Design review of the part built by this model. Coordinates are the model's own, in mm. Round coordinates to 2 decimals unless told otherwise and drop trailing zeros. Order: outer loops, then holes, each group sorted by start corner. A loop starts at its lowest first (then second) coordinate and runs counter-clockwise, first axis right, second up. Notation, with made-up numbers: M 51,81 L 85,81 A20 ccw 85,96 Z; hole C 76.5,-32 d9. An arc over 180 degrees is marked long. Use a Markdown table: item, result. Add a question column.
(1) Take a section at C-C (y = -57.48). Write out the cut boundary in (x, z), then the cut area to 3 significant figures.
(2) Take a section at D-D (x = 84). Write out the cut boundary in (y, z) (1 decimal).
(3) Take a section at B-B (y = 57.48). Write out the cut boundary in (x, z), then the cut area to 4 significant figures.
(4) To check wall thickness, follow probe 1 along Y at (x, z) = (94.45, 3.25) (3 decimals); probe 2 along Y at (x, z) = (95.75, 2.5) (3 decimals); probe 3 along Z at (x, y) = (88.5, 8.5). State the ranges of each line that lie inside material, in increasing order. Write a range as from..to.
(5) For pin 1 (5 mm diameter, centred on x = 94.5, z = 2, fed in from -Y) (3 decimals); pin 2 (8 mm diameter, centred on x = 90, z = -37.5, fed in from -Y); pin 3 (4 mm diameter, centred on x = 94.45, y = -57.48, fed in from -Z), all flat-tipped, find the tip position at first contact; note any pin that passes through.
(6) Take a section at A-A (x = 94.45). Write out the cut boundary in (y, z) (3 decimals), then the cut area to 3 significant figures.
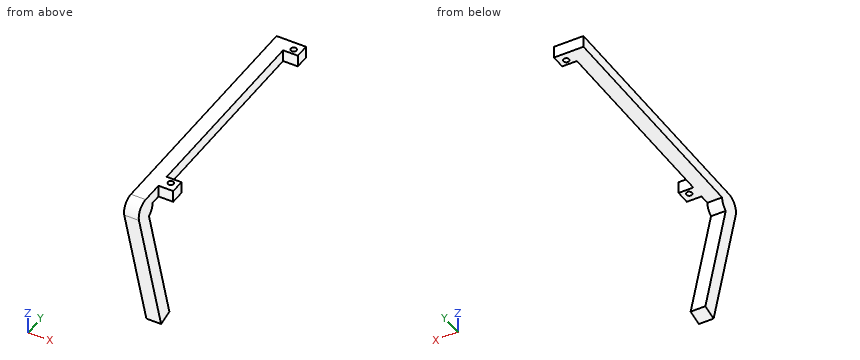
Autodesk Inventor part; units mm, degrees
ref_plane "YZ Plane" through (0, 0, 0) normal (1, 0, 0) x (0, 1, 0)
ref_plane "XZ Plane" through (0, 0, 0) normal (0, 1, 0) x (-1, 0, 0)
ref_plane "XY Plane" through (0, 0, 0) normal (0, 0, 1) x (1, 0, 0)
sketch "Sketch1" plane through (0, 0, 0) normal (0, 0, 1) x (1, 0, 0)
  line L0 (74.45, 62.135) -> (82.45, 62.135) construction
  line L1 (82.45, 62.135) -> (82.45, -62.135)
  line L2 (82.45, -62.135) -> (74.45, -62.135) construction
  circle A0 centre (78.45, 57.48) radius 1.55 construction
  circle A1 centre (78.45, -57.48) radius 1.55
  line L3 (78.45, 57.48) -> (78.45, -57.48) construction
  line L4 (74.45, 0) -> (82.45, 0) construction
  line L5 (74.45, 57.48) -> (82.45, 57.48) construction
  line L6 (74.45, 54.48) -> (82.45, 54.48) construction
  line L7 (74.45, -54.48) -> (82.45, -54.48) construction
  line L8 (82.45, 62.135) -> (90.45, 62.135)
  line L9 (90.45, 62.135) -> (90.45, -62.135)
  line L10 (90.45, -62.135) -> (82.45, -62.135)
  line L11 (82.45, -62.135) -> (82.45, 62.135)
  line L12 (74.45, -62.135) -> (74.45, -54.48) construction
  line L13 (74.45, 54.48) -> (74.45, 62.135) construction
  line L14 (74.45, 54.48) -> (74.45, -54.48) construction
  line L15 (0, 79.555) -> (0, -87.364) construction
  line L16 (74.45, -54.48) -> (82.45, -54.48) construction
  line L17 (82.45, -54.48) -> (82.45, -62.135)
  line L18 (82.45, -62.135) -> (74.45, -62.135) construction
  line L19 (74.45, -62.135) -> (74.45, -54.48) construction
  line L20 (86.45, 62.135) -> (86.45, -62.135) construction
  line L21 (98.45, 62.135) -> (90.45, 62.135)
  line L22 (90.45, 62.135) -> (90.45, -62.135)
  line L23 (90.45, -62.135) -> (98.45, -62.135)
  circle A2 centre (94.45, 57.48) radius 1.55
  circle A3 centre (94.45, -57.48) radius 1.55
  line L24 (98.45, 54.48) -> (90.45, 54.48)
  line L25 (98.45, -54.48) -> (90.45, -54.48)
  line L26 (98.45, 54.48) -> (98.45, 62.135)
  line L27 (98.45, -62.135) -> (98.45, -54.48)
  line L28 (90.45, -54.48) -> (90.45, -62.135)
  line L29 (90.45, -54.48) -> (98.45, -54.48)
  line L30 (98.45, -54.48) -> (98.45, -62.135)
  line L31 (98.45, -62.135) -> (90.45, -62.135)
  line L32 (90.45, -62.135) -> (90.45, -54.48)
  point P0 (0, 0)
  point P1 (78.45, 0)
  point P2 (78.45, 0)
  point P3 (78.45, 62.135)
  point P4 (78.45, -62.135)
  dimension "d0" = 124.27
  dimension "d1" = 8
  dimension "d2" = 3.1
  dimension "d3" = 3.1
  dimension "d4" = 114.96
  dimension "d5" = 3
  dimension "d6" = 78.45
  dimension "d7" = 8
extrude "Extrusion3" add sketch "Sketch1" along normal blind 6.5 contours L8 L9 L10 L1 | L21 L26 L24 L9 | L9 L25 L27 L23
sketch "Sketch4" plane through (90.45, -62.135, 0) normal (1, 0, 0) x (0, 0, -1)
  line L0 (-6.5, 7.655) -> (-6.5, 116.615)
  line L1 (-6.5, 0) -> (0, 0)
  line L2 (0, 0) -> (0, -12)
  line L3 (0, -12) -> (-6.5, -12)
  line L4 (-6.5, -12) -> (-6.5, 0)
  circle A0 centre (0, -12) radius 6.5
  line L5 (1.6823, -18.2785) -> (78.9564, 2.427)
  line L6 (78.9564, 2.427) -> (76.8858, 10.1544)
  line L7 (76.8858, 10.1544) -> (5.7208, -8.9142)
  point P0 (0, 62.135)
  point P1 (-7, 124.27)
  dimension "d19" = 12
  dimension "d20" = 75
  dimension "d21" = 8
  dimension "d22" = 80
extrude "Extrusion4" add sketch "Sketch4" against normal up to surface (8 mm away)
properties part number "LCD-holder-left"
Verdict:
| question | item | result |
|---|---|---|
| 1 | outline | M 82.45,-78.36 L 90.45,-78.36 L 90.45,-56.36 L 82.45,-56.36 Z; M 82.45,0 L 92.9,0 L 92.9,6.5 L 82.45,6.5 Z; M 96,0 L 98.45,0 L 98.45,6.5 L 96,6.5 Z |
| 1 | area | 260 mm^2 |
| 2 | outline | M -80.4,-1.7 L -59.7,-79 L -52,-76.9 L -71,-5.7 A6.5 ccw -67.6,0 L 62.1,0 L 62.1,6.5 L -74.1,6.5 A6.5 ccw Z |
| 3 | outline | M 82.45,0 L 92.9,0 L 92.9,6.5 L 82.45,6.5 Z; M 96,0 L 98.45,0 L 98.45,6.5 L 96,6.5 Z |
| 3 | area | 83.85 mm^2 |
| 4 | probe 1 | y = -62.135..-59.03, -55.93..-54.48, 54.48..55.93, 59.03..62.135 |
| 4 | probe 2 | y = -62.135..-58.324, -56.636..-54.48, 54.48..56.636, 58.324..62.135 |
| 4 | probe 3 | z = 0..6.5 |
| 5 | pin 1 | stops at y = -62.135 |
| 5 | pin 2 | stops at y = -71.89 |
| 5 | pin 3 | stops at z = 0 |
| 6 | outline | M -62.135,0 L -59.03,0 L -59.03,6.5 L -62.135,6.5 Z; M -55.93,0 L -54.48,0 L -54.48,6.5 L -55.93,6.5 Z; M 54.48,0 L 55.93,0 L 55.93,6.5 L 54.48,6.5 Z; M 59.03,0 L 62.135,0 L 62.135,6.5 L 59.03,6.5 Z |
| 6 | area | 59.2 mm^2 |
